Source: CAD feature listing. Evaluate the final solid. Frame: model axes, mm. A direction names the side the tool comes from. Coordinates: 2 decimals unless noted, no trailing zeros. Loops run counter-clockwise (first coordinate to the right, second up) from the corner with the lowest first, then second, coordinate; pieces in that order, holes last. Notation, with made-up numbers: (-11.5, 3) -> (-5.5, 3) arc R34 ccw to (-5.5, 35) -> close; hole circle Ø8 at (9.5, 20). An arc over 180 degrees is marked (long way). Answer as a JSON object with one key per item and string values. Group by question number.
from build123d import *

# Parameters (mm, degrees)
SKETCH1_R           = 23.85
BOSS_EXTRUDE1_DEPTH = 6
SKETCH2_R           = 25.5
BOSS_EXTRUDE2_DEPTH = 2
FILLET1_R           = 2
CUT_EXTRUDE1_DEPTH  = 37.939139135
BOSS_EXTRUDE3_DEPTH = 3
SKETCH5_W           = 28
SKETCH5_H           = 7.2
CUT_EXTRUDE2_DEPTH  = 3
SKETCH6_R           = 1.25
CUT_EXTRUDE3_DEPTH  = 5
FILLET2_R           = 2
CHAMFER1_SIZE       = 1
SKETCH7_W           = 1.25
SKETCH7_H           = 8


# Some blends are built 0.0001 mm under size
with BuildPart() as part:
    # Sketch1 → Boss-Extrude1 (new body)
    with BuildSketch(Plane(origin=(0, 0, 0), x_dir=(1, 0, 0), z_dir=(0, 1, 0))):
        with Locations(Location((0, 0, 0), (0, 0, 270))):
            Circle(SKETCH1_R)
    extrude(amount=BOSS_EXTRUDE1_DEPTH)

    # Sketch2 → Boss-Extrude2 (add)
    with BuildSketch(Plane(origin=(0, 6, 0), x_dir=(1, 0, 0), z_dir=(0, 1, 0))):
        with Locations(Location((0, 0, 0), (0, 0, 270))):
            Circle(SKETCH2_R)
    extrude(amount=BOSS_EXTRUDE2_DEPTH)

    # Fillet1
    fillet1_edges = [part.edges().sort_by_distance(p)[0] for p in [
        (0, 8, -25.5),
    ]]
    fillet(fillet1_edges, radius=FILLET1_R - 0.0001)  # a hair under: the kernel refuses the full size

    # Sketch3 → Cut-Extrude1 (cut, through all)
    with BuildSketch(Plane(origin=(0, 8, 0), x_dir=(1, 0, 0), z_dir=(0, 1, 0))):
        with BuildLine():
            Line((8.15, 0), (8.15, -7.5))
            ThreePointArc((8.15, -7.5), (0, -15.65), (-8.15, -7.5))
            Line((-8.15, -7.5), (-8.15, 0))
            ThreePointArc((-8.15, 0), (0, 8.15), (8.15, 0))
        make_face()
    extrude(amount=-CUT_EXTRUDE1_DEPTH, mode=Mode.SUBTRACT)

    # Sketch4 → Boss-Extrude3 (add)
    with BuildSketch(Plane.XZ):
        with BuildLine():
            Line((-12.15, 7.5), (-12.15, 0))
            ThreePointArc((-12.15, 0), (0, -12.15), (12.15, 0))
            Line((12.15, 0), (12.15, 7.5))
            ThreePointArc((12.15, 7.5), (0, 19.65), (-12.15, 7.5))
        make_face()
        with BuildLine():
            Line((8.15, 0), (8.15, 7.5))
            ThreePointArc((8.15, 7.5), (0, 15.65), (-8.15, 7.5))
            Line((-8.15, 7.5), (-8.15, 0))
            ThreePointArc((-8.15, 0), (0, -8.15), (8.15, 0))
        make_face(mode=Mode.SUBTRACT)
    extrude(amount=BOSS_EXTRUDE3_DEPTH)

    # Sketch5 → Cut-Extrude2 (cut)
    with BuildSketch(Plane.XZ.offset(3)):
        with Locations((0, 3.75)):
            Rectangle(SKETCH5_W, SKETCH5_H)
    extrude(amount=-CUT_EXTRUDE2_DEPTH, mode=Mode.SUBTRACT)

    # Sketch6 → Cut-Extrude3 (cut)
    with BuildSketch(Plane.XZ):
        with Locations(Location((-11, 3.75, 0), (0, 0, 270))):
            Circle(SKETCH6_R)
        with Locations(Location((11, 3.75, 0), (0, 0, 270))):
            Circle(SKETCH6_R)
    extrude(amount=-CUT_EXTRUDE3_DEPTH, mode=Mode.SUBTRACT)

    # Fillet2
    # the kernel refuses this fillet: 2 mm, written as the material it takes off along each edge
    with BuildSketch(Plane(origin=(8.15, -7.5749499, 0.15), x_dir=(-0.08318438898072168, 0, -0.9965341727356388), z_dir=(0, 1, 0)), Plane(origin=(8.15, 0, 7.35), x_dir=(-0.08318438898072168, 0, 0.9965341727356388), z_dir=(0, -1, 0)), Plane(origin=(-8.15, 0, 0.15), x_dir=(0.08318438898072168, 0, -0.9965341727356388), z_dir=(0, -1, 0)), Plane(origin=(-8.15, -7.5749499, 7.35), x_dir=(0.08318438898072159, 0, 0.9965341727356388), z_dir=(0, 1, 0))) as fillet2_piece_1:
        with BuildLine():
            CenterArc((1.840842581, -1.990006343), FILLET2_R, 95.730148145, 79.498223624)
            Line((-0.152225765, -1.823637565), (-0.351532599, -1.807000688))
            Line((-0.351532599, -1.807000688), (-0.199306835, 0.016636878))
            Line((-0.199306835, 0.016636878), (0.016636878, 0.199306835))
            ThreePointArc((0.016636878, 0.199306835), (0.166117004, 0.186829176), (1.62118728, 0.199000634))
            Line((1.62118728, 0.199000634), (1.641155943, 0))
        make_face()
    extrude(amount=7.5749499, mode=Mode.SUBTRACT)

    # Chamfer1
    chamfer1_edges = [part.edges().sort_by_distance(p)[0] for p in [
        (0, 8, -8.15),
        (-8.15, 8, 3.75),
        (0, 8, 15.65),
        (8.15, 8, 3.75),
    ]]
    chamfer(chamfer1_edges, length=CHAMFER1_SIZE)

    # Sketch7 → Cut-Revolve1 (revolve, cut)
    with BuildSketch(Plane(origin=(0, 3, 0), x_dir=(-1, 0, 0), z_dir=(0, -1, 0))):
        with Locations((0.625, -21.5)):
            Rectangle(SKETCH7_W, SKETCH7_H)
    revolve(axis=Axis((0, 3, 0), (0, 0, 1)), mode=Mode.SUBTRACT)


solid = part.part
1. Section query B-B on y = -2. Return loops of the section in (x, z), then the cut area to 3 significant figures.
2. Pin query (flat end, axial travel): pin 1 Ø1.1 at (x, y) = (11.5, -2) entering from +Z (3 decimals); pin 2 Ø4 at (x, y) = (1, -1) entering from +Z; pin 3 Ø1.1 at (x, y) = (-10.5, -2) entering from +Z; pin 4 Ø10 at (x, z) = (-15, 6) entering from -Y. Return the tip coordinate at first contact, or that it passes through.
3. Section query C-C on y = 3. Return loops of the section in (x, z).
4. Mould query, pull axis Z, two halves, no side actions, for faces 1 (the face through (-10, 8, 0)), 2 (the face through (7.16, 2.96, 22.75)), 3 (the face through (11, -2, 7.35)), 4 (the face through (-11, 5, 4)). Classes: pulls with the +Z half, pulls with the -Z half, needs draft (parallel to the pull), parting line crosses it, or undercut.
5. Reachability of faces 5 (the face through (-11, -2, 7.35)), 6 (the face through (0.18, 2.07, 15.65)), 7 (the face through (-0.18, 7.17, -8.32)), 8 (the face through (8.69, -1.48, 7.82)) from +Z, -Z, +X, -X, +Y, -Y: full face, straight path, thin tool, end or side. Return the list, or none.
6. Ray query, L1, parallel to X at y = 1.15, z = 3.75; L2, parallel to X at y = 5, z = 11; L3, parallel to Z at x = 3, y = -1. Return the intervals inside material, ascending.
Solved:
{
 "1": {"outline": "(-12.15, 0) arc R12.15 ccw to (12.15, 0) -> (12.15, 0.15) -> (9.98, 0.15) arc R2 ccw to (8.01, -1.49) arc R8.15 cw to (-8.01, -1.49) arc R2 ccw to (-9.98, 0.15) -> (-12.15, 0.15) -> close; (-12.15, 7.35) -> (-9.98, 7.35) arc R2 ccw to (-8.01, 8.99) arc R8.15 cw to (8.01, 8.99) arc R2 ccw to (9.98, 7.35) -> (12.15, 7.35) -> (12.15, 7.5) arc R12.15 ccw to (-12.15, 7.5) -> close", "area": "255 mm^2"},
 "2": {"pin 1": "z = 12.765", "pin 2": "z = 23.85", "pin 3": "z = 14.47", "pin 4": "y = -3"},
 "3": {"outline": "(-1.25, 17.5) -> (-1.25, 23.82) arc R23.85 ccw (long way) to (1.25, 23.82) -> (1.25, 17.5) -> close; hole circle Ø2.5 at (-11, 3.75); hole (-8.15, 0) arc R8.15 ccw to (8.15, 0) -> (8.15, 7.5) arc R8.15 ccw to (-8.15, 7.5) -> close; hole circle Ø2.5 at (11, 3.75)"},
 "4": {"face 1": "needs draft", "face 2": "parting line crosses it", "face 3": "undercut", "face 4": "undercut"},
 "5": {"face 5": "+X, -X, -Y", "face 6": "+Y, -Y", "face 7": "+Y", "face 8": "-Y"},
 "6": {"L1": "-23.55 to -12.25, -9.75 to -8.15, 8.15 to 9.75, 12.25 to 23.55", "L2": "-21.16 to -7.36, 7.36 to 21.16", "L3": "-11.77 to -7.58, 15.08 to 19.27"}
}
